Autodesk Inventor part; units mm, degrees
ref_plane "YZ Plane" through (0, 0, 0) normal (1, 0, 0) x (0, 1, 0)
ref_plane "XZ Plane" through (0, 0, 0) normal (0, 1, 0) x (-1, 0, 0)
ref_plane "XY Plane" through (0, 0, 0) normal (0, 0, 1) x (1, 0, 0)
sketch "Skizze9" plane through (0, 0, 0) normal (0, 1, 0) x (-1, 0, 0)
  line L0 (4.275, 15.405) -> (-4.275, 15.405)
  line L1 (-6.275, 13.405) -> (-6.275, -13.405)
  line L2 (-4.275, -15.405) -> (4.275, -15.405)
  line L3 (6.275, -13.405) -> (6.275, 13.405)
  line L4 (0, 0) -> (0, -15.405) construction
  line L5 (0, 0) -> (6.275, 0) construction
  arc A0 (6.275, 13.405) -> (4.275, 15.405) centre (4.275, 13.405) ccw
  arc A1 (-6.275, -13.405) -> (-4.275, -15.405) centre (-4.275, -13.405) ccw
  arc A2 (4.275, -15.405) -> (6.275, -13.405) centre (4.275, -13.405) ccw
  arc A3 (-4.275, 15.405) -> (-6.275, 13.405) centre (-4.275, 13.405) ccw
  point P0 (6.275, 15.405)
  point P1 (-6.275, -15.405)
  point P2 (-6.275, 15.405)
  point P3 (6.275, -15.405)
  dimension "d41" = 30.81
  dimension "d42" = 12.55
  dimension "d61" = 2
extrude "Extrusion6" add sketch "Skizze9" along normal blind 1
sketch "Skizze10" plane through (0, 1, 0) normal (0, 1, 0) x (1, 0, 0)
  line L0 (-4.275, -15.405) -> (4.275, -15.405)
  line L1 (6.275, -13.405) -> (6.275, 13.405)
  line L2 (4.275, 15.405) -> (-4.275, 15.405)
  line L3 (-6.275, 13.405) -> (-6.275, -13.405)
  line L4 (4.18, -5.3077) -> (4.18, 5.3077)
  line L5 (2.5273, 7.2773) -> (-1.8327, 8.0461)
  line L6 (-4.18, 6.0765) -> (-4.18, -6.0765)
  line L7 (-1.8327, -8.0461) -> (2.5273, -7.2773)
  line L8 (0, 0) -> (-4.18, 0) construction
  line L9 (0, 0) -> (4.18, 0) construction
  line L10 (-4.18, -8.46) -> (6.275, -8.46) construction
  line L11 (-4.18, 8.46) -> (6.275, 8.46) construction
  arc A0 (-4.18, -6.0765) -> (-1.8327, -8.0461) centre (-2.18, -6.0765) ccw
  arc A1 (-1.8327, 8.0461) -> (-4.18, 6.0765) centre (-2.18, 6.0765) ccw
  arc A2 (2.5273, -7.2773) -> (4.18, -5.3077) centre (2.18, -5.3077) ccw
  arc A3 (4.18, 5.3077) -> (2.5273, 7.2773) centre (2.18, 5.3077) ccw
  arc A4 (4.275, -15.405) -> (6.275, -13.405) centre (4.275, -13.405) ccw
  arc A5 (6.275, 13.405) -> (4.275, 15.405) centre (4.275, 13.405) ccw
  arc A6 (-4.275, 15.405) -> (-6.275, 13.405) centre (-4.275, 13.405) ccw
  arc A7 (-6.275, -13.405) -> (-4.275, -15.405) centre (-4.275, -13.405) ccw
  dimension "d45" = 10
  dimension "d46" = 4.18
  dimension "d47" = 4.18
  dimension "d48" = 16.92
  dimension "d49" = 2
extrude "Extrusion7" add sketch "Skizze10" along normal blind 6.1 contours A2 L7 A0 L6 A1 L5 A3 L4
sketch "Skizze11" plane through (0, 1, 0) normal (0, 1, 0) x (1, 0, 0)
  arc A0 (-1.8327, 8.0461) -> (-4.18, 6.0765) centre (-2.18, 6.0765) ccw
  line L0 (-1.8327, 8.0461) -> (2.5273, 7.2773)
  arc A1 (4.18, 5.3077) -> (2.5273, 7.2773) centre (2.18, 5.3077) ccw
  line L1 (4.18, 5.3077) -> (4.18, -5.3077)
  arc A2 (2.5273, -7.2773) -> (4.18, -5.3077) centre (2.18, -5.3077) ccw
  line L2 (2.5273, -7.2773) -> (-1.8327, -8.0461)
  arc A3 (-4.18, -6.0765) -> (-1.8327, -8.0461) centre (-2.18, -6.0765) ccw
  line L3 (-4.18, -6.0765) -> (-4.18, 6.0765)
  line L4 (-4.275, -15.405) -> (4.275, -15.405)
  line L5 (6.275, -13.405) -> (6.275, 13.405)
  line L6 (4.275, 15.405) -> (-4.275, 15.405)
  line L7 (-6.275, 13.405) -> (-6.275, -13.405)
  line L8 (0, 0) -> (0, 12.5) construction
  line L9 (0, 0) -> (0, -12.5) construction
  arc A4 (4.275, -15.405) -> (6.275, -13.405) centre (4.275, -13.405) ccw
  arc A5 (6.275, 13.405) -> (4.275, 15.405) centre (4.275, 13.405) ccw
  arc A6 (-4.275, 15.405) -> (-6.275, 13.405) centre (-4.275, 13.405) ccw
  arc A7 (-6.275, -13.405) -> (-4.275, -15.405) centre (-4.275, -13.405) ccw
  dimension "d52" = 12.5
  dimension "d53" = 12.5
hole "Bohrung3" at (0, 1, 12.5) at (0, 1, -12.5) direction (0, -1, 0) diameter 3.3 end through all
sketch "Skizze12" plane through (0, 0, 0) normal (0, -1, 0) x (1, 0, 0)
  circle A0 centre (0, 12.5) radius 1.65
  circle A1 centre (0, -12.5) radius 1.65
  line L0 (-4.275, 15.405) -> (4.275, 15.405)
  arc A2 (-4.275, 15.405) -> (-6.275, 13.405) centre (-4.275, 13.405) ccw
  line L1 (-6.275, -13.405) -> (-6.275, 13.405)
  arc A3 (-6.275, -13.405) -> (-4.275, -15.405) centre (-4.275, -13.405) ccw
  line L2 (4.275, -15.405) -> (-4.275, -15.405)
  arc A4 (4.275, -15.405) -> (6.275, -13.405) centre (4.275, -13.405) ccw
  line L3 (6.275, 13.405) -> (6.275, -13.405)
  arc A5 (6.275, 13.405) -> (4.275, 15.405) centre (4.275, 13.405) ccw
  line L4 (-5.3, -8.46) -> (5.3, -8.46)
  line L5 (5.3, -8.46) -> (5.3, 8.46)
  line L6 (5.3, 8.46) -> (-5.3, 8.46)
  line L7 (-5.3, 8.46) -> (-5.3, -8.46)
  line L8 (0, 0) -> (0, 8.46) construction
  line L9 (0, 0) -> (-5.3, 0) construction
  dimension "d62" = 10.6
  dimension "d63" = 16.92
extrude "Extrusion8" add sketch "Skizze12" along normal blind 12.5 contours L7 L6 L5 L4
properties part number "anschluss_daten_2"
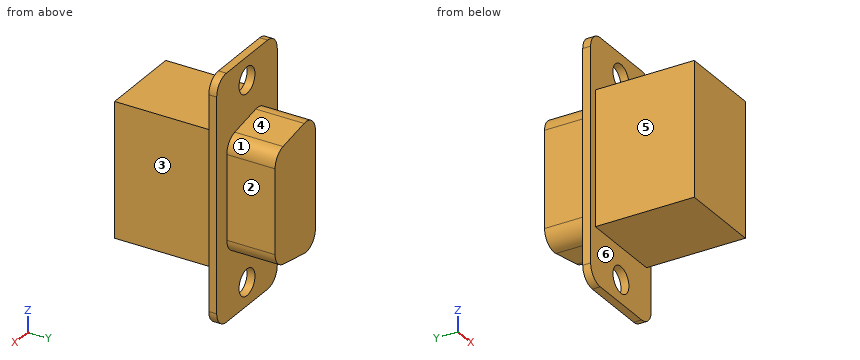
Design review of the part built by this model. Coordinates are the model's own, in mm. Face numbers are marked on the shaded views. A direction names the side the tool comes from. Round coordinates to 2 decimals unless told otherwise and drop trailing zeros. Write each loop counter-clockwise with the first axis right and the second up, starting at its lowest first coordinate (ties: lowest second). Pieces come first, ordered by that corner, then holes. Notation, with made-up numbers: (52, 29.5) -> (58, 29.5) arc R22 cw to (58, 45.5) -> close; hole circle Ø7 at (66.25, -34.75). An arc over 180 degrees is marked (long way). Write item = value, one per line. Start each with the question number.
1) Tool access review of the marked faces 1, 2 and 3: name each direction out of +Z, -Z, +X, -X, +Y, -Y from which nothing blocks a thin tool from reaching the whole face with its end or side.
2) Take a section at A-A, the plane y = 0.5. State the section outline as (x, z) points (3 decimals).
3) Take a section at B-B, the plane z = 12.5. State the section outline as (x, y) points (3 decimals).
4) Take a section at C-C, the plane x = 0. State the section outline as (y, z) points (3 decimals), plus the area to 3 significant figures.
5) Mouldability with a two-part tool opening along X and no side actions: class the marked faces 4, 5 and 6 as +X half, -X half, draft (parallel to the pull), parting line (faces both ways), or undercut.
6) Clearance check with flat-ended pins moving along their axes: pin 1 (3 mm diameter, centred on x = 2, y = -2.5, fed in from +Z); pin 2 (2 mm diameter, centred on x = 4.5, y = 3, fed in from +Z); pin 3 (5 mm diameter, centred on y = 4.5, z = 1, fed in from +X). State where each tip first meets the part, or that it passes through.
7) Take a section at D-D, the plane z = -1.5. State the section outline as (x, y) points (3 decimals), plus the area to 3 significant figures.
8) Wall thickness on probe 1 along Z at (x, y) = (0, 0.7) (3 decimals); probe 2 along X at (y, z) = (0.2, -12.5) (3 decimals); probe 3 along Y at (x, z) = (-4.5, -8): over which ranges is each line inside the solid? List them lowest first. Write a range as from..to.
Results list:
q1.face_1 = +Z, +X, +Y
q1.face_2 = +Z, -Z, +X, +Y
q1.face_3 = +Z, -Z, +X, -Y
q2.outline = (-6.275, -13.405) arc R2 ccw to (-4.275, -15.405) -> (4.275, -15.405) arc R2 ccw to (6.275, -13.405) -> (6.275, 13.405) arc R2 ccw to (4.275, 15.405) -> (-4.275, 15.405) arc R2 ccw to (-6.275, 13.405) -> close; hole circle Ø3.3 at (0, -12.5); hole circle Ø3.3 at (0, 12.5)
q3.outline = (-6.275, 0) -> (-1.65, 0) -> (-1.65, 1) -> (-6.275, 1) -> close; (1.65, 0) -> (6.275, 0) -> (6.275, 1) -> (1.65, 1) -> close
q4.outline = (-12.5, -8.46) -> (0, -8.46) -> (0, -10.85) -> (1, -10.85) -> (1, -7.723) -> (7.1, -7.723) -> (7.1, 7.723) -> (1, 7.723) -> (1, 10.85) -> (0, 10.85) -> (0, 8.46) -> (-12.5, 8.46) -> close; (0, -15.405) -> (1, -15.405) -> (1, -14.15) -> (0, -14.15) -> close; (0, 14.15) -> (1, 14.15) -> (1, 15.405) -> (0, 15.405) -> close
q4.area = 330 mm²
q5.face_4 = +X half
q5.face_5 = -X half
q5.face_6 = draft
q6.pin_1 = 8.46
q6.pin_2 = 6.81
q6.pin_3 = 4.18
q7.outline = (-6.275, 0) -> (-5.3, 0) -> (-5.3, -12.5) -> (5.3, -12.5) -> (5.3, 0) -> (6.275, 0) -> (6.275, 1) -> (4.18, 1) -> (4.18, 7.1) -> (-4.18, 7.1) -> (-4.18, 1) -> (-6.275, 1) -> close
q7.area = 196 mm²
q8.probe_1 = -15.405..-14.15, -10.85..10.85, 14.15..15.405
q8.probe_2 = -6.275..-1.65, 1.65..6.275
q8.probe_3 = -12.5..1
